Verification items for the finished model (mm, model axes). A direction names the side the tool comes from. Coordinates: 2 decimals unless noted, no trailing zeros. Order: outer loops, then holes, each group sorted by start corner. A loop starts at its lowest first (then second) coordinate and runs counter-clockwise, first axis right, second up. Notation, with made-up numbers: M 85.25,85.25 L 142.25,85.25 A9 cw 142.25,91.25 Z; hole C -17,-22 d3. An arc over 180 degrees is marked long. Return JSON: item names as keys, results as strings.
```python
from build123d import *

# Parameters (mm, degrees)
F0_R     = 76.2
F0_R_2   = 36.5125
F1_DEPTH = 9.525
F2_W     = 4.7625
F2_H     = 30.1625
F3_DEPTH = 47.625
F4_SIZE  = 4.445
F6_D     = 11.1125
F7_R     = 5.08
F8_SIZE  = 0.635


with BuildPart() as f1:
    # F0 (on Top) → F1 (new body)
    with BuildSketch(Plane.XY):
        Circle(F0_R)
        with BuildLine():
            Line((-22.680412, -43.370582), (-30.145285, -53.645098))
            ThreePointArc((-30.145285, -53.645098), (-40.123691, -55.225523), (-41.704115, -45.247117))
            Line((-41.704115, -45.247117), (-34.239242, -34.972601))
            ThreePointArc((-34.239242, -34.972601), (-24.260836, -33.392176), (-22.680412, -43.370582))
        make_face(mode=Mode.SUBTRACT)
        with BuildLine():
            ThreePointArc((7.14375, -61.11875), (0, -68.2625), (-7.14375, -61.11875))
            Line((-7.14375, -61.11875), (-7.14375, -48.41875))
            ThreePointArc((-7.14375, -48.41875), (0, -41.275), (7.14375, -48.41875))
            Line((7.14375, -48.41875), (7.14375, -61.11875))
        make_face(mode=Mode.SUBTRACT)
        with BuildLine():
            Line((34.239242, -34.972601), (41.704115, -45.247117))
            ThreePointArc((41.704115, -45.247117), (40.123691, -55.225523), (30.145285, -53.645098))
            Line((30.145285, -53.645098), (22.680412, -43.370582))
            ThreePointArc((22.680412, -43.370582), (24.260836, -33.392176), (34.239242, -34.972601))
        make_face(mode=Mode.SUBTRACT)
        with BuildLine():
            ThreePointArc((-61.11875, -7.14375), (-68.2625, 0), (-61.11875, 7.14375))
            Line((-61.11875, 7.14375), (-48.41875, 7.14375))
            ThreePointArc((-48.41875, 7.14375), (-41.275, 0), (-48.41875, -7.14375))
            Line((-48.41875, -7.14375), (-61.11875, -7.14375))
        make_face(mode=Mode.SUBTRACT)
        with BuildLine():
            Line((-48.256508, 8.168107), (-60.334926, 12.092622))
            ThreePointArc((-60.334926, 12.092622), (-64.921495, 21.094273), (-55.919845, 25.680842))
            Line((-55.919845, 25.680842), (-43.841428, 21.756327))
            ThreePointArc((-43.841428, 21.756327), (-39.254858, 12.754676), (-48.256508, 8.168107))
        make_face(mode=Mode.SUBTRACT)
        Circle(F0_R_2, mode=Mode.SUBTRACT)
        with BuildLine():
            ThreePointArc((61.11875, 7.14375), (68.2625, 0), (61.11875, -7.14375))
            Line((61.11875, -7.14375), (48.41875, -7.14375))
            ThreePointArc((48.41875, -7.14375), (41.275, 0), (48.41875, 7.14375))
            Line((48.41875, 7.14375), (61.11875, 7.14375))
        make_face(mode=Mode.SUBTRACT)
        with BuildLine():
            Line((43.841428, 21.756327), (55.919845, 25.680842))
            ThreePointArc((55.919845, 25.680842), (64.921495, 21.094273), (60.334926, 12.092622))
            Line((60.334926, 12.092622), (48.256508, 8.168107))
            ThreePointArc((48.256508, 8.168107), (39.254858, 12.754676), (43.841428, 21.756327))
        make_face(mode=Mode.SUBTRACT)
        with BuildLine():
            ThreePointArc((-7.14375, 61.11875), (0, 68.2625), (7.14375, 61.11875))
            Line((7.14375, 61.11875), (7.14375, 48.41875))
            ThreePointArc((7.14375, 48.41875), (0, 41.275), (-7.14375, 48.41875))
            Line((-7.14375, 48.41875), (-7.14375, 61.11875))
        make_face(mode=Mode.SUBTRACT)
    extrude(amount=F1_DEPTH)

    # F2 (on face) → F3 (join)
    with BuildSketch(Plane.XY.offset(9.525)):
        with Locations((38.89375, 48.971965)):
            Rectangle(F2_W, F2_H)
        with Locations((-38.89375, 48.971965)):
            Rectangle(F2_W, F2_H)
    extrude(amount=F3_DEPTH)

    # F4
    f4_edges = [f1.edges().sort_by_distance(p)[0] for p in [
        (-36.5125, 0, 0),
    ]]
    chamfer(f4_edges, length=F4_SIZE)

    # F6 (through all)
    with Locations(Plane.YZ.offset(41.275)):
        with Locations((48.971965, 46.83125)):
            Hole(F6_D / 2)

    # F7
    f7_edges = [f1.edges().sort_by_distance(p)[0] for p in [
        (38.89375, 33.890715, 57.15),
        (38.89375, 64.053215, 57.15),
        (-38.89375, 33.890715, 57.15),
        (-38.89375, 64.053215, 57.15),
    ]]
    fillet(f7_edges, radius=F7_R)

    # F8
    f8_edges = [f1.edges().sort_by_distance(p)[0] for p in [
        (-36.5125, 0, 9.525),
    ]]
    chamfer(f8_edges, length=F8_SIZE)


solid = f1.part
```
Q1. Material ranges on line 1 along Y through (x, z) = (0, 5.9) (1 decimal); line 2 along X through (y, z) = (46.5, 17.5) (1 decimal); line 3 along X through (y, z) = (-3, 8.5), recorded low to high.
Values:
{"line 1": "-76.2 to -68.3, -41.3 to -36.5, 36.5 to 41.3, 68.3 to 76.2", "line 2": "-41.3 to -36.5, 36.5 to 41.3", "line 3": "-76.14 to -67.6, -41.94 to -36.39, 36.39 to 41.94, 67.6 to 76.14"}
Q2. Cross-section at A-A, the plane z = 38. Record the boundary of the cut face in (x, y) (1 decimal).
Values:
{"outline": "M -41.3,33.9 L -36.5,33.9 L -36.5,64.1 L -41.3,64.1 Z; M 36.5,33.9 L 41.3,33.9 L 41.3,64.1 L 36.5,64.1 Z"}
Q3. Draft check along X on faces 3 (the face through (55, 7.144, 5)), 4 (the face through (41.275, 49, 33)), 5 (the face through (-38.86, 62.605, 55.622)), 6 (the face through (-64.97, 20.94, 4.7)). Enter one of: pulls with the +X half, pulls with the -X half, needs draft (parallel to the pull), parting line crosses it, or undercut.
Values:
{"face 3": "undercut", "face 4": "pulls with the +X half", "face 5": "needs draft", "face 6": "undercut"}
Q4. Tool access check on faces 1 (the face through (-39, 49, 57.15)), 2 (the face through (-7.144, -55, 5)). Record the directions out of +Z, -Z, +X, -X, +Y, -Y that give a thin tool (end or side, any length) a straight path to the whole face; none if there is none.
Values:
{"face 1": "+Z, +X, -X, +Y, -Y", "face 2": "+Z, -Z"}
Q5. Cross-section at B-B, the plane x = 0. State how many separate pieces and enclosed holes the cut face has, and give its area (3 significant figures).
Values:
{"separate pieces": "4", "enclosed holes": "0", "area": "222 mm^2"}
Q6. Go/stop test with flat-tipped pins: pin 1 (4 mm diameter, centred on x = -39.5, z = 38, fed in from +Y); pin 2 (9 mm diameter, centred on y = 54.5, z = 36.5, fed in from +X) (3 decimals); pin 3 (10.5 mm diameter, centred on x = 56, z = 5, fed in from -Y). Record where each tip stops, or that it passes through.
Values:
{"pin 1": "y = 64.05", "pin 2": "x = 41.275", "pin 3": "y = -56.84"}
